from build123d import *

# Parameters (mm, degrees)
SKETCH_1_W      = 28
SKETCH_1_H      = 28
SKETCH_1_R      = 1.25
EXTRUDE_1_DEPTH = 41
SKETCH_2_R      = 10
EXTRUDE_2_DEPTH = 3
SKETCH_3_R      = 2.5
EXTRUDE_3_DEPTH = 20
FILLET_1_R      = 2


with BuildPart() as part:
    # 草图1 → 凸台-拉伸1 (new body)
    with BuildSketch(Plane.XY):
        Rectangle(SKETCH_1_W, SKETCH_1_H)
        with Locations((-11.5, 11.5)):
            Circle(SKETCH_1_R, mode=Mode.SUBTRACT)
        with Locations((11.5, 11.5)):
            Circle(SKETCH_1_R, mode=Mode.SUBTRACT)
        with Locations((11.5, -11.5)):
            Circle(SKETCH_1_R, mode=Mode.SUBTRACT)
        with Locations((-11.5, -11.5)):
            Circle(SKETCH_1_R, mode=Mode.SUBTRACT)
    extrude(amount=EXTRUDE_1_DEPTH)

    # 草图2 → 凸台-拉伸2 (add)
    with BuildSketch(Plane.XY.offset(41)):
        Circle(SKETCH_2_R)
    extrude(amount=EXTRUDE_2_DEPTH)

    # 草图3 → 凸台-拉伸3 (add)
    with BuildSketch(Plane.XY.offset(44)):
        Circle(SKETCH_3_R)
    extrude(amount=EXTRUDE_3_DEPTH)

    # 圆角1
    fillet_1_edges = [part.edges().sort_by_distance(p)[0] for p in [
        (14, -14, 20.5),
        (-14, -14, 20.5),
        (-14, 14, 20.5),
        (14, 14, 20.5),
    ]]
    fillet(fillet_1_edges, radius=FILLET_1_R)


solid = part.part
CAD build for the part. Positions are in the model's coordinates, mm. A direction names the side the tool comes from. Coordinates: 2 decimals unless noted, no trailing zeros. Order: outer loops, then holes, each group sorted by start corner. A loop starts at its lowest first (then second) coordinate and runs counter-clockwise, first axis right, second up.
Item 1: 3-axis set-ups, long thin cutter, end or side, ignore diameter. For faces 1 (the face through (10.579, -10.655, 20.213)), 2 (the face through (2, -2, 44)): which of +Z, -Z, +X, -X, +Y, -Y reach the whole face in a straight line?
Check sheet entries:
face 1: +Z, -Z
face 2: +Z
Item 2: Band-saw the part on C-C on z = 54. List the corners of the cut face in (x, y), plus the area to 3 significant figures.
Check sheet entries:
outline: circle Ø5 at (0, 0)
area: 19.6 mm2
Item 3: Band-saw the part on A-A on y = 0. List the corners of the cut face in (x, z).
Check sheet entries:
outline: (-14, 0) - (14, 0) - (14, 41) - (10, 41) - (10, 44) - (2.5, 44) - (2.5, 64) - (-2.5, 64) - (-2.5, 44) - (-10, 44) - (-10, 41) - (-14, 41) - close
Item 4: Drill centre lines: L1, parallel to Y at x = 11.5, z = 24; L2, parallel to X at y = 10.5, z = 32; L3, parallel to X at y = -12.5, z = 6. Where is each one in solid material? Low to high.
Check sheet entries:
L1: y = -14 to -12.75, -10.25 to 10.25, 12.75 to 14
L2: x = -14 to -12.25, -10.75 to 10.75, 12.25 to 14
L3: x = -13.94 to -12.25, -10.75 to 10.75, 12.25 to 13.94
Item 5: Band-saw the part on D-D on x = 11. List the corners of the cut face in (y, z), plus the area to 3 significant figures.
Check sheet entries:
outline: (-14, 0) - (-12.65, 0) - (-12.65, 41) - (-14, 41) - close; (-10.35, 0) - (10.35, 0) - (10.35, 41) - (-10.35, 41) - close; (12.65, 0) - (14, 0) - (14, 41) - (12.65, 41) - close
area: 960 mm2
Item 6: Pin check, flat tips, straight feed: pin 1 Ø1.5 at (x, y) = (-1.5, 8.5) entering from +Z; pin 2 Ø4 at (x, y) = (-11.5, -11.5) entering from +Z. Stop position of each tip, or through.
Check sheet entries:
pin 1: stops at z = 44
pin 2: stops at z = 41
Item 7: Two-plate mould, pull along Y, no slides. Class faces 3 (the face through (-12.421, 12.345, 20.213)), 4 (the face through (-13.43, -13.4, 20.79)), 5 (the face through (14, 0, 20)): +Y half, -Y half, draft (parallel to the pull), parting line (faces both ways), or undercut.
Check sheet entries:
face 3: undercut
face 4: -Y half
face 5: draft
